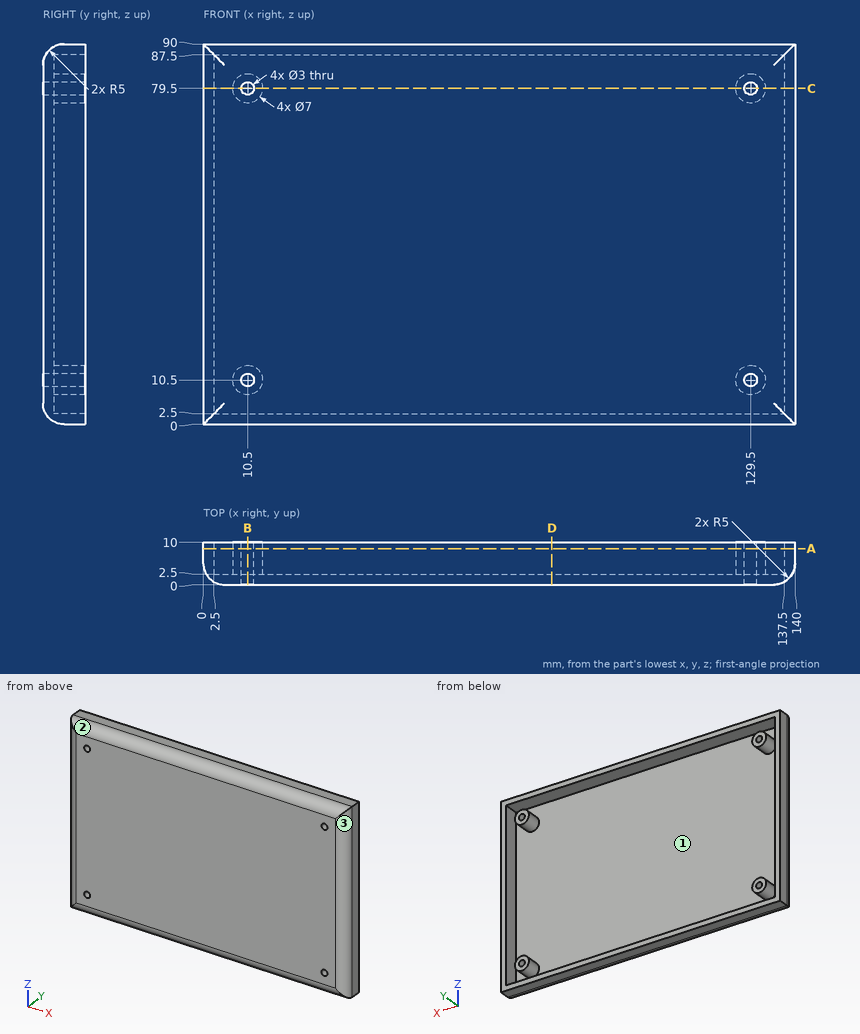
Geometry check sheet. Reference: drawing and pictorial views, mm from the part's lowest x, y, z. Give positions to 0.01 mm unless a question says otherwise; leave off trailing zeros. Write each loop counter-clockwise with the first axis right and the second up, starting at its lowest first coordinate (ties: lowest second). Pieces come first, ordered by that corner, then holes. Notation, with made-up numbers: (37, 25) -> (56, 25) arc R23 cw to (56, 42) -> close; hole circle Ø6 at (66.5, -6.75). An arc over 180 degrees is marked (long way). One line per question, with ' | ' between items.
Item 1: Scan lines: line 1 along X through (y, z) = (6.75, 79.5); line 2 along X through (y, z) = (7.5, 73); line 3 along X through (y, z) = (4.75, 8). Record each from-to range of solid material in increasing order.
Determined:
line 1: 0 to 2.5, 7 to 9, 12 to 14, 126 to 128, 131 to 133, 137.5 to 140 | line 2: 0 to 2.5, 137.5 to 140 | line 3: 0.01 to 2.5, 8.05 to 12.95, 127.05 to 131.95, 137.5 to 139.99
Item 2: Sectioned sample at B-B, the plane x = 10.5. Record the boundary of the cut face in (y, z), plus the area to 3 significant figures.
Determined:
outline: (0, 5) arc R5 ccw to (5, 0) -> (10, 0) -> (10, 2.5) -> (2.5, 2.5) -> (2.5, 7) -> (10, 7) -> (10, 9) -> (0, 9) -> close; (0, 12) -> (10, 12) -> (10, 14) -> (2.5, 14) -> (2.5, 76) -> (10, 76) -> (10, 78) -> (0, 78) -> close; (0, 81) -> (10, 81) -> (10, 83) -> (2.5, 83) -> (2.5, 87.5) -> (10, 87.5) -> (10, 90) -> (5, 90) arc R5 ccw to (0, 85) -> close | area: 297 mm^2
Item 3: Sectioned sample at A-A, the plane y = 8.5. State how many separate pieces and enclosed holes the cut face has, plus the area to 3 significant figures.
Determined:
separate pieces: 5 | enclosed holes: 5 | area: 1,250 mm^2
Item 4: Sectioned sample at D-D, the plane x = 82.5. Record the boundary of the cut face in (y, z), plus the area to 3 significant figures.
Determined:
outline: (0, 5) arc R5 ccw to (5, 0) -> (10, 0) -> (10, 2.5) -> (2.5, 2.5) -> (2.5, 87.5) -> (10, 87.5) -> (10, 90) -> (5, 90) arc R5 ccw to (0, 85) -> close | area: 252 mm^2
Item 5: Sectioned sample at C-C, the plane z = 79.5. Record the boundary of the cut face in (x, y), plus the area to 3 significant figures.
Determined:
outline: (0, 5) arc R5 ccw to (5, 0) -> (9, 0) -> (9, 10) -> (7, 10) -> (7, 2.5) -> (2.5, 2.5) -> (2.5, 10) -> (0, 10) -> close; (12, 0) -> (128, 0) -> (128, 10) -> (126, 10) -> (126, 2.5) -> (14, 2.5) -> (14, 10) -> (12, 10) -> close; (131, 0) -> (135, 0) arc R5 ccw to (140, 5) -> (140, 10) -> (137.5, 10) -> (137.5, 2.5) -> (133, 2.5) -> (133, 10) -> (131, 10) -> close | area: 422 mm^2
Item 6: Draft check along X on the marked faces 1, 2 and 3. Enter one of: released by +X, released by -X, zero draft, split by the parting line, or undercut.
Determined:
face 1: undercut | face 2: zero draft | face 3: released by +X
Item 7: Depth check by flat-ended pin: pin 1 (8 mm diameter, centred on x = 35, z = 42.5, fed in from +Y); pin 2 (1.8 mm diameter, centred on x = 129.5, z = 10.5, fed in from +Y); pin 3 (3.5 mm diameter, centred on x = 10.5, z = 79.5, fed in from +Y); pin 4 (1 mm diameter, centred on x = 30, y = 3.5, fed in from -Z). Enter the tip coordinate at first touch or a pass-through.
Determined:
pin 1: y = 2.5 | pin 2: through | pin 3: y = 10 | pin 4: z = 0.1
